Read the model definition and answer for the solid it produces. Units are mm, in the model's axes. Face numbers are marked on the shaded views. Give positions to 0.01 mm unless a question says otherwise; leave off trailing zeros. Order: outer loops, then holes, each group sorted by start corner. A loop starts at its lowest first (then second) coordinate and runs counter-clockwise, first axis right, second up. Notation, with made-up numbers: (26, 78) - (53, 78) arc R15 ccw to (53, 93) - close; hole circle Ø4 at (42.25, 21.25). An arc over 180 degrees is marked (long way). Write each question's results on one line, items separated by ' | '. Start each with the question number.
Q1. For a pull along Y with two mould halves and no side action, classify the marked faces 1 and 2 as +Y half, -Y half, draft (parallel to the pull), parting line (faces both ways), or undercut.
Q2. Find section A-A on x = 50. Give the vertices of the cut face in (y, z), and give its area (3 significant figures).
Q3. Find the intervals of material crossed by line 1 along Y through (x, z) = (38.5, 25.5); line 2 along Y through (x, z) = (74.5, 3.5); line 3 along X through (y, z) = (35.5, 19.5), in increasing order. Write a range as from..to.
Q4. Find section B-B on z = 11. Count the separate pieces of the cut face and the enclosed holes in it, and give its area (3 significant figures).
Q5. Find section C-C on y = 9.5. Give the vertices of the cut face in (x, z).
Q6. Find section D-D on x = 25. Give the vertices of the cut face in (y, z).
Q7. A flat-ended cylindrical pin translates along its axis: P1, Ø4, axis at x = 9.5, y = 38.5, coming from the +Z side. Find the tip coordinate at first contact, or state that the pin passes through.
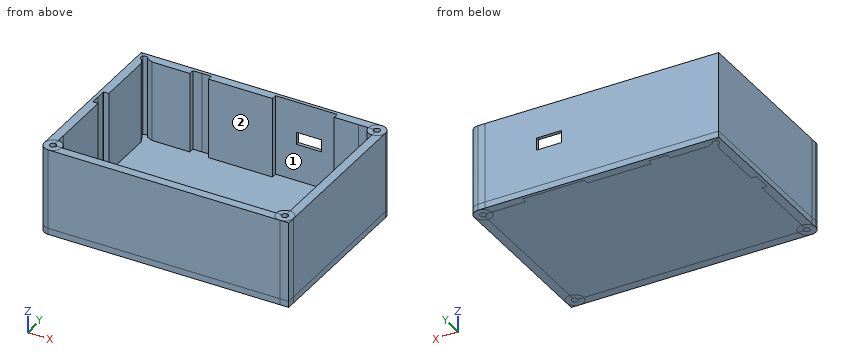
Autodesk Fusion 360 part; units mm, degrees
sketch "Sketch1" plane through (0, 0, 0) normal (0, 0, 1) x (1, 0, 0)
  line L0 (0, 0.9105) -> (0, 44.7087)
  line L1 (2.2913, 47) -> (17.5, 47)
  line L2 (17.5, 47) -> (15.35, 47)
  line L3 (0, 23.5) -> (0, 25.65)
  line L4 (0, 23.5) -> (0, 21.35)
  line L5 (-1.7, 23.5) -> (-1.7, 25.8)
  line L6 (-1.7, 23.5) -> (-1.7, 21.2)
  line L7 (70, 47) -> (74, 47) construction
  line L8 (0, 47) -> (-2.8284, 49.8284)
  line L9 (0, 47) -> (-4, 47) construction
  line L10 (-2.8284, 49.8284) -> (72.8284, 49.8284)
  line L11 (-2.8284, 49.8284) -> (-2.8284, -2.8284)
  line L12 (17.5, 47) -> (69, 47)
  line L13 (41.1957, 48.7475) -> (61.1957, 48.7475)
  line L14 (41.1957, 48.7475) -> (41.1957, 47)
  line L15 (61.1957, 48.7475) -> (61.1957, 47)
  line L16 (17.5, 48.7) -> (14.5, 48.7)
  line L17 (14.5, 48.7) -> (20.5, 48.7)
  line L18 (20.5, 48.7) -> (20.5, 47)
  line L19 (14.5, 48.7) -> (14.5, 47)
  line L20 (-1.7, 23.5) -> (-1.7, 26.5)
  line L21 (-1.7, 26.5) -> (-1.7, 23.5)
  line L22 (-1.7, 23.5) -> (-1.7, 20.5)
  line L23 (-1.7, 20.5) -> (-1.7, 26.5)
  line L24 (0, 26.5) -> (-1.7, 26.5)
  line L25 (-1.7, 20.5) -> (0, 20.5)
  line L26 (0, 47) -> (0, 48)
  line L27 (0, 48) -> (2.2913, 47)
  line L28 (0, 47) -> (-1, 47)
  line L29 (-1, 47) -> (0, 44.7087)
  arc A0 (0, 48) -> (-1, 47) centre (0, 47) ccw
  line L30 (-2.8284, 49.8284) -> (-2.8284, -7.8286)
  line L31 (-2.8284, 49.8284) -> (77.8286, 49.8284)
  line L32 (77.8286, 49.8284) -> (77.8286, -7.8286)
  line L33 (77.8286, -7.8286) -> (-2.8284, -7.8286)
  line L34 (0, -5) -> (75, -5)
  line L35 (75, -5) -> (75, 47)
  line L36 (75, 47) -> (69, 47)
  line L37 (0, 0.9105) -> (0, -5)
  circle A1 centre (75, 47) radius 2.8284
  circle A2 centre (75, 47) radius 1.05
  circle A3 centre (75, -5) radius 2.8286
  circle A4 centre (75, -5) radius 1.05
  circle A5 centre (0, -5) radius 2.8284
  circle A6 centre (0, -5) radius 1.05
  circle A7 centre (-0.7071, 47.7071) radius 1.05
  dimension "d2" = 47
  dimension "d3" = 17.5
  dimension "d5" = 2.15
  dimension "d23" = 2.15
  dimension "d25" = 1.7
  dimension "d26" = 2.3
  dimension "d27" = 2.3
  dimension "d33" = 45
  dimension "d34" = 4
  dimension "d59" = 6
  dimension "d60" = 3
  dimension "d61" = 3
  dimension "d63" = 2
  dimension "d70" = 20
  dimension "d72" = 2.5
  dimension "d73" = 2.5
  dimension "d126" = 57.657
  dimension "d127" = 80.657
  dimension "d128" = 2.1
  dimension "d129" = 2.1
  dimension "d130" = 2.1
  dimension "d131" = 2.1
sketch "Sketch2" plane through (0, 49.8284, 0) normal (0, 1, 0) x (-1, 0, 0)
  line L0 (-72.8284, 0) -> (2.8284, 0)
  line L1 (2.8284, 0) -> (2.8284, 28)
  line L2 (2.8284, 28) -> (-72.8284, 28)
  line L3 (-72.8284, 28) -> (-72.8284, 0)
  line L4 (-72.8284, 0) -> (-42.8284, 0)
  line L5 (-42.8284, 0) -> (-52.0284, 0)
  line L6 (-52.0284, 0) -> (-52.0284, 18)
  line L7 (-52.0284, 18) -> (-56.0284, 18)
  line L8 (-56.0284, 18) -> (-48.0284, 18)
  line L9 (-48.0284, 18) -> (-48.0284, 15)
  line L10 (-56.0284, 15) -> (-56.0284, 18)
  line L11 (-56.0284, 18) -> (-48, 18)
  line L12 (-48, 18) -> (-48, 14)
  line L13 (-48, 14) -> (-56.0284, 14)
  line L14 (-56.0284, 14) -> (-56.0284, 18)
  dimension "d49" = 30
  dimension "d50" = 9.2
  dimension "d51" = 18
  dimension "d52" = 4
  dimension "d53" = 8
  dimension "d54" = 3
extrude "Extrude25" add sketch "Sketch1" along normal blind 28 contours L0 L5 L6 L8 L11 L20 L21 L22 L23 L24 L25 L29 L30 L37 A5 A7 | L34 L37 A5 A6 | L34 L37 A5 A6 | L33 L34 A3 A5 | L34 L35 A3 A4 | L34 L35 A3 A4 | L32 L35 A1 A3 | L32 L33 A3 | L1 L8 L10 L12 L13 L14 L15 L16 L17 L18 L19 L27 L31 L36 A1 A7 | L35 L36 A1 A2 | L35 L36 A1 A2
extrude "Extrude26" add sketch "Sketch1" along normal blind 2 contours L0 L5 L6 L8 L11 L20 L21 L22 L23 L24 L25 L29 L30 L37 A5 A7 | L0 L1 L2 L3 L4 L12 L27 L29 L34 L35 L36 L37 A1 A3 A5 A7 | L0 L3 L4 L5 L6 L20 L21 L22 L23 L24 L25 | L34 L37 A5 A6 | L34 L37 A5 A6 | L34 L37 A6 | L34 L37 A6 | L33 L34 A3 A5 | L34 L35 A3 A4 | L34 L35 A3 A4 | L34 L35 A4 | L34 L35 A4 | L32 L35 A1 A3 | L32 L33 A3 | L1 L8 L10 L12 L13 L14 L15 L16 L17 L18 L19 L27 L31 L36 A1 A7 | L35 L36 A1 A2 | L35 L36 A1 A2 | L8 L27 A0 A7 | L8 L29 A0 A7 | L35 L36 A2 | L35 L36 A2 | L8 L26 A0 | L8 L28 A0 | L26 L27 L28 L29 A7 | L12 L13 L14 L15 | L1 L2 L12 L16 L17 L18 L19
extrude "Extrude27" cut sketch "Sketch2" against normal blind 6 contours L6 L7 L8 L10 L11 L13 L14 | L6 L8 L11 L12 L13
equation "d3 = ( 35 / 2 ) * 1 mm"
equation "d50 = ( 18.4 / 2 ) * 1 mm"
Working result:
1) face 1: undercut | face 2: undercut
2) outline: (-7.83, 0) - (49.83, 0) - (49.83, 14) - (48.75, 14) - (48.75, 2) - (-5, 2) - (-5, 28) - (-7.83, 28) - close; (48.75, 18) - (49.83, 18) - (49.83, 28) - (48.75, 28) - close | area: 213 mm²
3) line 1: -7.83..-5, 47..49.83 | line 2: -7.83..-5.92, -4.08..-2.22, 44.22..46.08, 47.92..49.83 | line 3: -2.83..0, 75..77.83
4) separate pieces: 1 | enclosed holes: 4 | area: 695 mm²
5) outline: (-2.83, 0) - (77.83, 0) - (77.83, 28) - (75, 28) - (75, 2) - (0, 2) - (0, 28) - (-2.83, 28) - close
6) outline: (-7.83, 0) - (49.83, 0) - (49.83, 28) - (47, 28) - (47, 2) - (-5, 2) - (-5, 28) - (-7.83, 28) - close
7) P1: z = 2
